from build123d import *

# Parameters (mm, degrees)
BOSS_EXTRUDE1_START = 6.35
SKETCH3_R           = 7.9375
SKETCH3_R_2         = 4.7752
BOSS_EXTRUDE1_DEPTH = 1.5875
BOSS_EXTRUDE2_START = 4.7625
SKETCH4_R           = 6.3627
SKETCH4_R_2         = 4.7752
BOSS_EXTRUDE2_DEPTH = 11.1125
CHAMFER1_SIZE       = 0.143256


with BuildPart() as part:
    # Sketch3 → Boss-Extrude1 (new body)
    with BuildSketch(Plane.XY.offset(BOSS_EXTRUDE1_START)):
        Circle(SKETCH3_R)
        Circle(SKETCH3_R_2, mode=Mode.SUBTRACT)
    extrude(amount=-BOSS_EXTRUDE1_DEPTH)

    # Sketch4 → Boss-Extrude2 (add)
    with BuildSketch(Plane.XY.offset(BOSS_EXTRUDE2_START)):
        Circle(SKETCH4_R)
        Circle(SKETCH4_R_2, mode=Mode.SUBTRACT)
    extrude(amount=-BOSS_EXTRUDE2_DEPTH)

    # Chamfer1
    chamfer1_edges = [part.edges().sort_by_distance(p)[0] for p in [
        (-4.7752, 0, -6.35),
        (-6.3627, 0, 4.7625),
        (-7.9375, 0, 6.35),
        (-7.9375, 0, 4.7625),
        (-4.7752, 0, 6.35),
        (-6.3627, 0, -6.35),
    ]]
    chamfer(chamfer1_edges, length=CHAMFER1_SIZE)


solid = part.part
CAD build for the part. Positions are in the model's coordinates, mm. A direction names the side the tool comes from. Coordinates: 2 decimals unless noted, no trailing zeros. Write each loop counter-clockwise with the first axis right and the second up, starting at its lowest first coordinate (ties: lowest second). Pieces come first, ordered by that corner, then holes. Notation, with made-up numbers: (3, -21) - (60, -21) arc R28 ccw to (60, 4) - close; hole circle Ø6 at (-40, -8.5). An arc over 180 degrees is marked (long way). Use a Markdown table: item, result. Add a question column.
Item 1: Mould opens along Y. For faces 3 (the face through (5.1, 0.1, 6.35)), 4 (the face through (-1.04, -4.66, 0.09)), 5 (the face through (-0.83, 6.31, -0.72)) say: pulls with the +Y half, pulls with the -Y half, needs draft (parallel to the pull), parting line crosses it, or undercut.
Item 2: Band-saw the part on A-A, the plane y = 0. Give the cut face in (x, z), and give its area (3 significant figures).
Item 3: 3-axis set-ups, long thin cutter, end or side, ignore diameter. For faces 1 (the face through (5, 2, -6.35)), 2 (the face through (-5, -5, 4.762)): which of +Z, -Z, +X, -X, +Y, -Y reach the whole face in a straight line?
Item 4: Flat gauge pins, fed straight in: pin 1 (3 mm diameter, centred on x = 6, z = -4.5, fed in from -Y); pin 2 (2 mm diameter, centred on x = 6.5, y = -6, fed in from -Z); pin 3 (1.5 mm diameter, centred on x = 0.5, z = -1.5, fed in from +Y). Where does each tip first touch, or does it go through?
Item 5: Drill centre lines: L1, parallel to Y at x = 0, z = 1; L2, parallel to Z at x = -5.5, y = -3.5; L3, parallel to X at y = 4.25, z = 2.5. Where is each one in solid material? Low to high. Write a range as from..to.
Item 6: Band-saw the part on C-C, the plane z = 2.5. Give the cut face in (x, y).
Numbers:
| question | item | result |
|---|---|---|
| 1 | face 3 | needs draft |
| 1 | face 4 | undercut |
| 1 | face 5 | parting line crosses it |
| 2 | outline | (-7.94, 4.91) - (-7.79, 4.76) - (-6.51, 4.76) - (-6.36, 4.62) - (-6.36, -6.21) - (-6.22, -6.35) - (-4.92, -6.35) - (-4.78, -6.21) - (-4.78, 6.21) - (-4.92, 6.35) - (-7.79, 6.35) - (-7.94, 6.21) - close; (4.78, -6.21) - (4.92, -6.35) - (6.22, -6.35) - (6.36, -6.21) - (6.36, 4.62) - (6.51, 4.76) - (7.79, 4.76) - (7.94, 4.91) - (7.94, 6.21) - (7.79, 6.35) - (4.92, 6.35) - (4.78, 6.21) - close |
| 2 | area | 45.2 mm2 |
| 3 | face 1 | -Z, +X, -X, +Y, -Y |
| 3 | face 2 | -Z |
| 4 | pin 1 | y = -4.5 |
| 4 | pin 2 | z = 4.81 |
| 4 | pin 3 | y = 6.36 |
| 5 | L1 | -6.36..-4.78, 4.78..6.36 |
| 5 | L2 | 4.76..6.35 |
| 5 | L3 | -4.74..-2.18, 2.18..4.74 |
| 6 | outline | circle Ø12.73 at (0, 0); hole circle Ø9.55 at (0, 0) |
